Part model, mm, in its own coordinate system. Face numbers are marked on the shaded views. Give positions to 0.01 mm unless a question says otherwise; leave off trailing zeros. Order: outer loops, then holes, each group sorted by start corner. A loop starts at its lowest first (then second) coordinate and runs counter-clockwise, first axis right, second up.
1. Mould opens along X. For the marked faces 1 and 2 say: +X half, -X half, draft (parallel to the pull), parting line (faces both ways), or undercut.
2. Drop flat-ended pins along their axis: pin 1 Ø8 at (y, z) = (-15.5, 33.5) entering from -X; pin 2 Ø1 at (y, z) = (-13, 23) entering from -X; pin 3 Ø12 at (x, y) = (-18, -19.5) entering from -Z. Give the stop position or say it passes through.
3. Probe line 1 (X direction, y = -5.75, z = 26); line 2 (Z direction, x = -17, y = -8.5); line 3 (X direction, y = -5.5, z = 1.5). List the from-to ranges inside material, lowest first.
4. Slice it at C-C on y = -23. List the corners of the cut face in (x, z).
5. Slice it at B-B on y = -8.5. List the corners of the cut face in (x, z).
6. Slice it at A-A on z = 0. List the corners of the cut face in (x, y).
from build123d import *

# Parameters (mm, degrees)
F0_R     = 46.157486
F1_DEPTH = 25
F3_DEPTH = 25
F4_R     = 10


with BuildPart() as f1:
    # F0 (on Front) → F1 (new body)
    with BuildSketch(Plane.XZ):
        Circle(F0_R)
    extrude(amount=F1_DEPTH)

    # F2 (on face) → F3 (cut)
    with BuildSketch(Plane.XZ.offset(25)):
        Polygon((0, 26.293665), (-20.571175, -13.729163), (19.424781, -14.297934), align=None)
    extrude(amount=-F3_DEPTH, mode=Mode.SUBTRACT)

    # F4
    f4_edges = [f1.edges().sort_by_distance(p)[0] for p in [
        (-46.157486, -25, 0),
        (-46.157486, 0, 0),
    ]]
    fillet(f4_edges, radius=F4_R)


solid = f1.part
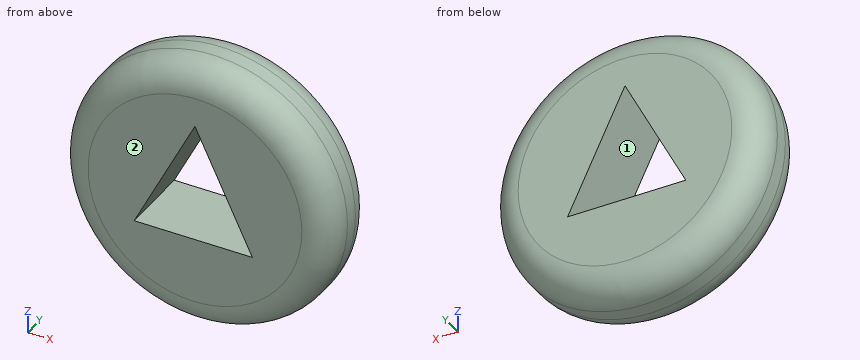
Data:
1. face 1: undercut
1. face 2: draft
2. pin 1: stops at x = -35.49
2. pin 2: stops at x = -40.3
2. pin 3: stops at z = -44.23
3. line 1: x = -36.99 to -0.15, 0.14 to 36.99
3. line 2: z = -42.79 to -13.78, -6.78 to 42.79
3. line 3: x = -45.06 to -12.74, 11.86 to 45.06
4. outline: circle Ø84.31 at (0, 0); hole (-20.57, -13.73) - (19.42, -14.3) - (0, 26.29) - close
5. outline: circle Ø92.09 at (0, 0); hole (-20.57, -13.73) - (19.42, -14.3) - (0, 26.29) - close
6. outline: (-46.16, -15) arc R10 ccw to (-36.16, -25) - (-13.51, -25) - (-13.51, 0) - (-36.16, 0) arc R10 ccw to (-46.16, -10) - close; (12.58, -25) - (36.16, -25) arc R10 ccw to (46.16, -15) - (46.16, -10) arc R10 ccw to (36.16, 0) - (12.58, 0) - close
